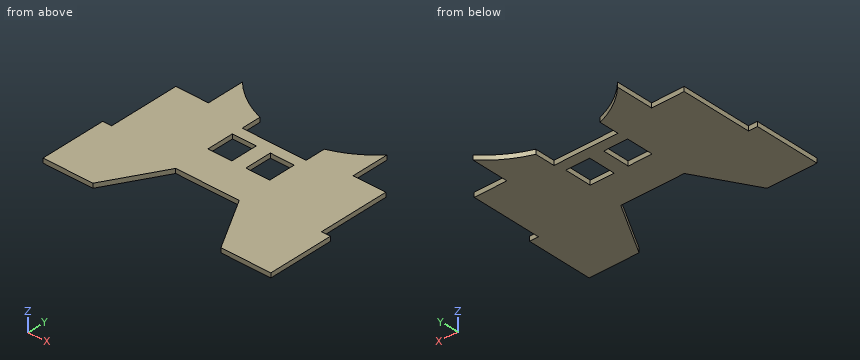
from build123d import *

# Parameters (mm, degrees)
BOSS_EXTRUDE1_DEPTH = 5
SKETCH2_W           = 26.358753283
SKETCH2_H           = 29.759882739
CUT_EXTRUDE1_DEPTH  = 5
SKETCH3_W           = 34.735720487
SKETCH3_H           = 8.029761026
BOSS_EXTRUDE2_DEPTH = 5
SKETCH4_W           = 54.614047871
SKETCH4_H           = 63
SKETCH4_W_2         = 55.31958059
CUT_EXTRUDE2_DEPTH  = 10


with BuildPart() as part:
    # Sketch1 → Boss-Extrude1 (new body)
    with BuildSketch(Plane.XY):
        with BuildLine():
            Line((-91.993742522, 102.725612705), (-126.729463009, 102.725612705))
            Line((-126.729463009, 102.725612705), (-126.746200519, 82.983777967))
            Line((-126.746200519, 82.983777967), (-126.751305113, 69.550155563))
            Line((-126.751305113, 69.550155563), (-126.751615017, 54.928897922))
            Line((-126.751615017, 54.928897922), (-116.909086823, 54.928897922))
            Line((-116.909086823, 54.928897922), (-116.909086823, -30.41815046))
            Line((-116.909086823, -30.41815046), (-126.752882712, -30.41815046))
            Line((-126.752882712, -30.41815046), (-126.752882712, -102.974632312))
            Line((-126.752882712, -102.974632312), (-71.719920422, -102.974632312))
            Line((-71.719920422, -102.974632312), (-36.199181634, -41.450908009))
            Line((-36.199181634, -41.450908009), (33.804891756, -41.450908009))
            Line((33.804891756, -41.450908009), (69.325630544, -102.974632312))
            Line((69.325630544, -102.974632312), (124.358592834, -102.974632312))
            Line((124.358592834, -102.974632312), (124.358592834, -30.41815046))
            Line((124.358592834, -30.41815046), (114.641773971, -30.41815046))
            ThreePointArc((114.641773971, -30.41815046), (114.551987655, -30.38095975), (114.514796945, -30.291173434))
            Line((114.514796945, -30.291173434), (114.514796945, 54.801920897))
            ThreePointArc((114.514796945, 54.801920897), (114.551987655, 54.891707213), (114.641773971, 54.928897922))
            Line((114.641773971, 54.928897922), (124.357325139, 54.928897922))
            Line((124.357325139, 54.928897922), (124.357015448, 69.54009331))
            Line((124.357015448, 69.54009331), (124.351902115, 82.993834667))
            Line((124.351902115, 82.993834667), (124.335173131, 102.725612705))
            Line((124.335173131, 102.725612705), (89.599452644, 102.725612705))
            ThreePointArc((89.599452644, 102.725612705), (65.571107836, 77.403597365), (34.818671263, 60.885320824))
            Line((34.818671263, 60.885320824), (34.818671263, 38.755373731))
            Line((34.818671263, 38.755373731), (-35.581655871, 38.755373731))
            Line((-35.581655871, 38.755373731), (-35.581655871, 60.334309069))
            ThreePointArc((-35.581655871, 60.334309069), (-67.279163206, 76.883706742), (-91.993742522, 102.725612705))
        make_face()
    extrude(amount=BOSS_EXTRUDE1_DEPTH)

    # Sketch2 → Cut-Extrude1 (cut)
    with BuildSketch(Plane.XY.offset(5)):
        with Locations((19.127528046, 12.255373732)):
            Rectangle(SKETCH2_W, SKETCH2_H)
        with Locations((-22.712961142, 12.255373732)):
            Rectangle(SKETCH2_W, SKETCH2_H)
    extrude(amount=-CUT_EXTRUDE1_DEPTH, mode=Mode.SUBTRACT)

    # Sketch3 → Boss-Extrude2 (add)
    with BuildSketch(Plane.XY.offset(5)):
        with Locations((-109.361602766, 106.740493218)):
            Rectangle(SKETCH3_W, SKETCH3_H)
        with Locations((106.967312888, 106.740493218)):
            Rectangle(SKETCH3_W, SKETCH3_H)
    extrude(amount=-BOSS_EXTRUDE2_DEPTH)

    # Sketch4 → Cut-Extrude2 (cut)
    with BuildSketch(Plane.XY.offset(5)):
        with Locations((105.82182088, 79.255373731)):
            Rectangle(SKETCH4_W, SKETCH4_H)
        with Locations((-108.568877118, 79.255373731)):
            Rectangle(SKETCH4_W_2, SKETCH4_H)
    extrude(amount=-CUT_EXTRUDE2_DEPTH, mode=Mode.SUBTRACT)


solid = part.part
Part model, mm, in its own coordinate system. Round coordinates to 2 decimals unless told otherwise and drop trailing zeros. Order: outer loops, then holes, each group sorted by start corner. A loop starts at its lowest first (then second) coordinate and runs counter-clockwise, first axis right, second up. Notation, with made-up numbers: (15.25, 48.25) -> (44.25, 48.25) arc R33 ccw to (44.25, 79.25) -> close; hole circle Ø10 at (24, 82). An arc over 180 degrees is marked (long way). Put each result on its own line as item: value.
Q1. Pin check, flat tips, straight feed: pin 1 Ø1.5 at (x, z) = (16, 3) entering from -Y; pin 2 Ø2.5 at (x, z) = (24.5, 3.5) entering from +Y; pin 3 Ø1.5 at (x, z) = (-107, 2) entering from +Y. Stop position of each tip, or through.
From the geometry:
pin 1: stops at y = -41.45
pin 2: stops at y = 38.76
pin 3: stops at y = 47.76
Q2. Band-saw the part on A-A (y = 45). Give the cut face in (x, z), and give its area (3 significant figures).
From the geometry:
outline: (-116.91, 0) -> (-35.58, 0) -> (-35.58, 5) -> (-116.91, 5) -> close; (34.82, 0) -> (114.51, 0) -> (114.51, 5) -> (34.82, 5) -> close
area: 805 mm2
Q3. Band-saw the part on C-C (x = 22). Give the cut face in (y, z).
From the geometry:
outline: (-41.45, 0) -> (-2.62, 0) -> (-2.62, 5) -> (-41.45, 5) -> close; (27.14, 0) -> (38.76, 0) -> (38.76, 5) -> (27.14, 5) -> close
Q4. Band-saw the part on D-D (y = 24.5). Give the cut face in (x, z).
From the geometry:
outline: (-116.91, 0) -> (-35.89, 0) -> (-35.89, 5) -> (-116.91, 5) -> close; (-9.53, 0) -> (5.95, 0) -> (5.95, 5) -> (-9.53, 5) -> close; (32.31, 0) -> (114.51, 0) -> (114.51, 5) -> (32.31, 5) -> close
Q5. Wall check: line 1 (X direction, y = 55.5, z = 0.9); line 2 (Y direction, x = -13, z = 2.3); line 3 (X direction, y = 6, z = 2.1). Give the ranges that are in metal, low to high. Write a range as [from, to].
From the geometry:
line 1: x = [-80.91, -35.58], [34.82, 78.51]
line 2: y = [-41.45, -2.62], [27.14, 38.76]
line 3: x = [-116.91, -35.89], [-9.53, 5.95], [32.31, 114.51]
Q6. Band-saw the part on B-B (z = 2.4). State how many separate pieces and enclosed holes the cut face has, and give its area (3 significant figures).
From the geometry:
separate pieces: 1
enclosed holes: 2
area: 29,800 mm2
